Drawing for the job (mm, zero at the part's lowest x, y, z). Coordinates: 2 decimals unless noted, no trailing zeros. Write each loop counter-clockwise with the first axis right and the second up, starting at its lowest first coordinate (ties: lowest second). Pieces come first, ordered by that corner, then holes. Notation, with made-up numbers: M 88,36.25 L 113,36.25 A24 ccw 113,73.25 Z; hole C 86.5,-35 d11. An arc over 180 degrees is marked long. Put each result on its own line as item: value. Start each with the question number.
Q1. Pull direction Y, two halves, no side cores. Call the marked faces 1, 2 and 3: pulls with the +Y half, pulls with the -Y half, needs draft (parallel to the pull), parting line crosses it, or undercut.
Q2. Cut at B-B (y = 9.25). Write the cut outline in (x, z).
Q3. Cut at A-A (z = 41.5). Write the cut outline in (x, y).
Q4. Cut at C-C (x = 93). Write the cut outline in (y, z), then the cut area to 3 significant figures.
Q5. Drill centre lines: line 1 along Y through (x, z) = (18, 28.5); line 2 along Y through (x, z) = (81, 94); line 3 along X through (y, z) = (10.25, 33.5). Where is each one in solid material? Low to high.
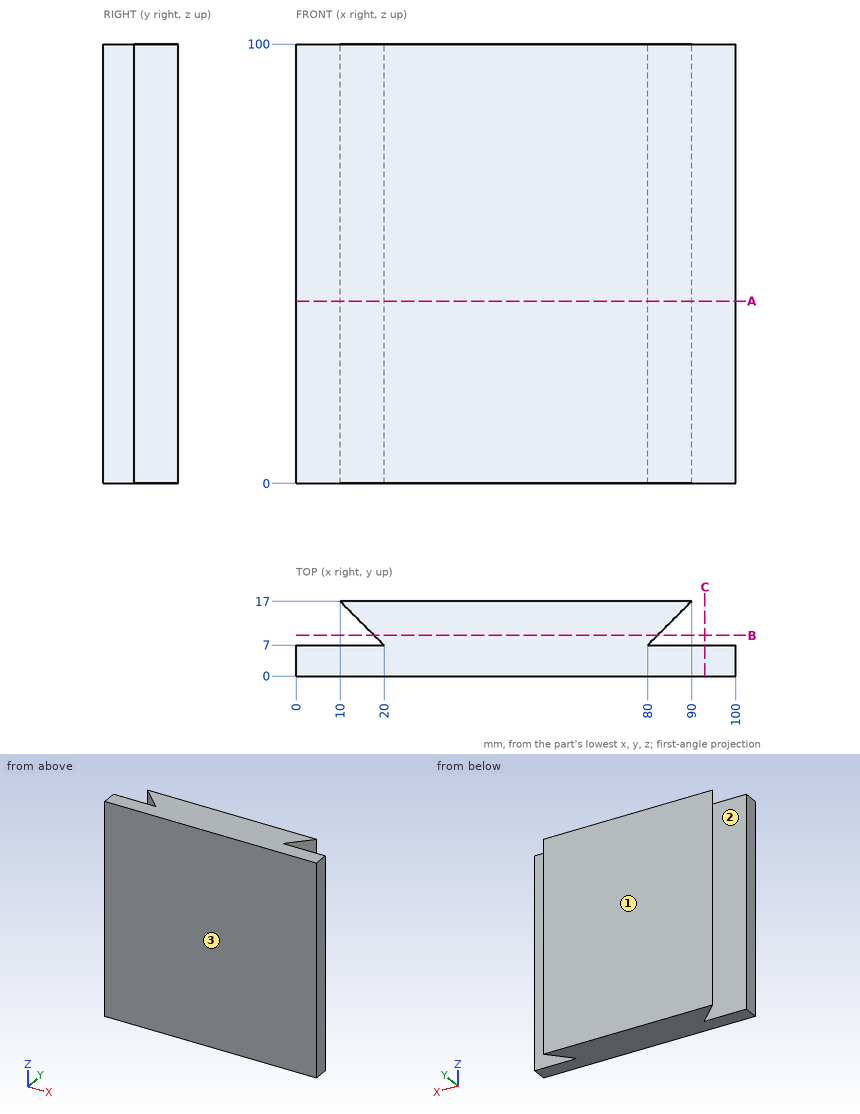
Computed values:
1. face 1: pulls with the +Y half
1. face 2: undercut
1. face 3: pulls with the -Y half
2. outline: M 17.75,0 L 82.25,0 L 82.25,100 L 17.75,100 Z
3. outline: M 0,0 L 100,0 L 100,7 L 80,7 L 90,17 L 10,17 L 20,7 L 0,7 Z
4. outline: M 0,0 L 7,0 L 7,100 L 0,100 Z
4. area: 700 mm2
5. line 1: 0 to 7, 9 to 17
5. line 2: 0 to 7, 8 to 17
5. line 3: 16.75 to 83.25
